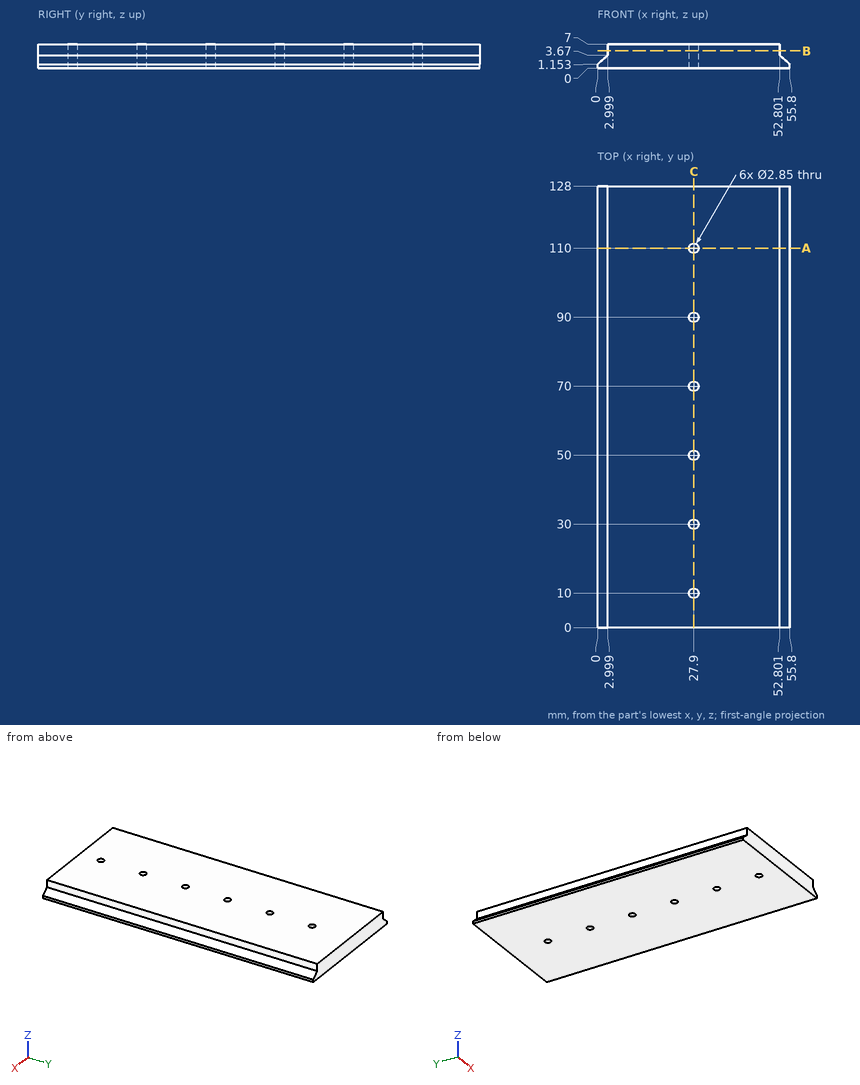
Source: three-view drawing plus pictorial views. Frame: mm from the lowest corner of the part. Give positions to 0.01 mm unless a question says otherwise; leave off trailing zeros. Order: outer loops, then holes, each group sorted by start corner. A loop starts at its lowest first (then second) coordinate and runs counter-clockwise, first axis right, second up. Notation, with made-up numbers: (-14, 30.25) -> (-4, 30.25) arc R28 cw to (-4, 51.25) -> close; hole circle Ø7 at (-11.75, -1.75). An arc over 180 degrees is marked (long way). Use a Markdown table: item, result.
Q1. Section C-C (x = 27.9). Return the cut outline in (y, z) (1 decimal).
A:
| item | result |
|---|---|
| outline | (0, 0) -> (8.6, 0) -> (8.6, 7) -> (0, 7) -> close; (11.4, 0) -> (28.6, 0) -> (28.6, 7) -> (11.4, 7) -> close; (31.4, 0) -> (48.6, 0) -> (48.6, 7) -> (31.4, 7) -> close; (51.4, 0) -> (68.6, 0) -> (68.6, 7) -> (51.4, 7) -> close; (71.4, 0) -> (88.6, 0) -> (88.6, 7) -> (71.4, 7) -> close; (91.4, 0) -> (108.6, 0) -> (108.6, 7) -> (91.4, 7) -> close; (111.4, 0) -> (128, 0) -> (128, 7) -> (111.4, 7) -> close |
Q2. Section A-A (y = 110). Return the cut outline in (x, z) (1 decimal).
A:
| item | result |
|---|---|
| outline | (0, 0) -> (26.5, 0) -> (26.5, 7) -> (3, 7) -> (3, 3.7) -> (0, 1.2) -> close; (29.3, 0) -> (55.8, 0) -> (55.8, 1.2) -> (52.8, 3.7) -> (52.8, 7) -> (29.3, 7) -> close |
Q3. First-contact query: P1, Ø2.5, axis at y = 34, z = 4.5, coming from the -X side; P2, Ø1, axis at y = 86, z = 5, coming from the +X side. Flat tips, straight axial feed; report the tip coordinate or a pass-through.
A:
| item | result |
|---|---|
| P1 | x = 2.5 |
| P2 | x = 52.8 |
Q4. Section B-B (z = 5). State how many separate pieces and enclosed holes the cut face has, and give its area (3 significant figures).
A:
| item | result |
|---|---|
| separate pieces | 1 |
| enclosed holes | 6 |
| area | 6,340 mm^2 |
Q5. Material intervals for line 1 (X direction, y = 10, z = 5.75) (1 decimal); line 2 (X direction, y = 34.5, z = 6.75); line 3 (X direction, y = 110, z = 3.5) (1 decimal), sorted ascending. Write a range as [from, to].
A:
| item | result |
|---|---|
| line 1 | [3, 26.5], [29.3, 52.8] |
| line 2 | [3, 52.8] |
| line 3 | [2.8, 26.5], [29.3, 53] |
